Autodesk Fusion 360 part; units mm, degrees
sketch "Sketch1" plane through (0, 0, 0) normal (0, 0, 1) x (1, 0, 0)
  line L0 (0, 0) -> (20.646, 0)
  line L1 (20.646, 0) -> (20.646, 50)
  line L2 (20.646, 50) -> (0, 50)
  line L3 (0, 50) -> (0, 0)
  dimension "d1" = 20.646
  dimension "d2" = 50
extrude "Extrude1" add sketch "Sketch1" along normal blind 5
sketch "Sketch2" plane through (0, 0, 5) normal (0, 0, 1) x (-1, 0, 0)
  line L0 (0, -50) -> (0, 0)
  line L1 (0, 0) -> (-20.646, 0)
  line L2 (-20.646, 0) -> (-20.646, -50)
  line L3 (-20.646, -50) -> (0, -50)
sketch "Sketch3" plane through (0, 0, 5) normal (0, 0, 1) x (-1, 0, 0)
  line L0 (-20.646, 0) -> (-20.646, -50)
  line L1 (0, -50) -> (0, 0)
  circle A0 centre (-10.323, -25) radius 8.0085
  dimension "d5" = 16.017
extrude "Extrude2" cut sketch "Sketch3" against normal blind 10
sketch "Sketch4" plane through (0, 0, 5) normal (0, 0, 1) x (-1, 0, 0)
  circle A0 centre (-10.323, -25) radius 8.0085
  line L0 (-10.323, -25) -> (-2.3221, -33.0009)
  line L1 (-10.323, -25) -> (-2.3221, -16.9991)
  line L2 (-10.323, -25) -> (-18.3239, -16.9991)
  line L3 (-10.323, -25) -> (-18.3239, -33.0009)
hole "Hole1" at (2.3221, 16.9991, 5) at (2.3221, 33.0009, 5) at (18.3239, 33.0009, 5) at (18.3239, 16.9991, 5) direction (0, 0, -1) diameter 1.623 depth 16 tip angle 180 counterbore diameter 3.9 counterbore depth 1
sketch "Sketch5" plane through (0, 0, 5) normal (0, 0, 1) x (-1, 0, 0)
  circle A0 centre (-2.3221, -33.0009) radius 1.95
  line L0 (-2.3221, -33.0009) -> (-2.3221, -44.0009)
  circle A1 centre (-18.3239, -33.0009) radius 1.95
  line L1 (-18.3239, -33.0009) -> (-18.3239, -44.0009)
  circle A2 centre (-2.3221, -16.9991) radius 1.95
  line L2 (-2.3221, -16.9991) -> (-2.3221, -5.9991)
  circle A3 centre (-18.3239, -16.9991) radius 1.95
  line L3 (-18.3239, -16.9991) -> (-18.3239, -5.9991)
  dimension "d16" = 11
  dimension "d17" = 11
  dimension "d18" = 11
  dimension "d19" = 11
hole "Hole2" at (2.3221, 5.9991, 5) at (18.3239, 5.9991, 5) at (18.3239, 44.0009, 5) at (2.3221, 44.0009, 5) direction (0, 0, -1) diameter 1.623 end through all counterbore diameter 3.9 counterbore depth 1
sketch "Sketch6" plane through (0, 0, 5) normal (0, 0, 1) x (-1, 0, 0)
Here's how the part is built. I have some questions about the finished solid (model axes, mm). A direction names the side the tool comes from. Give positions to 0.01 mm unless a question says otherwise; leave off trailing zeros. Write each loop counter-clockwise with the first axis right and the second up, starting at its lowest first coordinate (ties: lowest second). Pieces come first, ordered by that corner, then holes.
(1) If I drill on L1, parallel to Y at x = 10.5, z = 4.7; L2, parallel to X at y = 33.5, z = 0.3; L3, parallel to Y at x = 1.25, z = 4.2, over which ranges is the centre line in solid material (lowest first)?
Output values:
L1: y = 0 to 16.99, 33.01 to 50
L2: x = 0 to 1.68, 2.96 to 17.68, 18.96 to 20.65
L3: y = 0 to 4.37, 7.63 to 15.37, 18.63 to 31.37, 34.63 to 42.37, 45.63 to 50
(2) On a 3-axis mill with a long thin cutter (end or side, diameter ignored), from which of +Z, -Z, +X, -X, +Y, -Y can I reach the whole of each face in a straight line? I mean faces 4 (the face through (2, 32, 4)), 5 (the face through (18.82, 17.64, 1.97)). Say none if no direction works.
Output values:
face 4: +Z
face 5: +Z, -Z
(3) Imagine slicing it at B-B, the plane z = 1.1. Count the separate pieces of the cut face and the enclosed holes in it, and give its area (3 significant figures).
Output values:
separate pieces: 1
enclosed holes: 9
area: 814 mm2
(4) Thinking about a two-plate mould opening in Y: for faces 1 (the face through (2, 43, 4)), 2 (the face through (10, 50, 2)), 3 (the face through (10, 0, 2)), which applies, pulls with the +Y half, pulls with the -Y half, needs draft (parallel to the pull), parting line crosses it, or undercut?
Output values:
face 1: undercut
face 2: pulls with the +Y half
face 3: pulls with the -Y half
(5) Imagine slicing it at A-A, the plane y = 25. Write out the boundary of the cut face in (x, z).
Output values:
outline: (0, 0) - (2.31, 0) - (2.31, 5) - (0, 5) - close; (18.33, 0) - (20.65, 0) - (20.65, 5) - (18.33, 5) - close
(6) Will these pins go through, and if not, where does the flat tip stop? pin 1 (2.5 mm diameter, centred on x = 18.32, y = 44, fed in from +Z); pin 2 (1 mm diameter, centred on x = 2.32, y = 17, fed in from -Z).
Output values:
pin 1: stops at z = 4
pin 2: passes through
(7) Imagine slicing it at C-C, the plane x = 9.5. Write out the boundary of the cut face in (y, z).
Output values:
outline: (0, 0) - (17.03, 0) - (17.03, 5) - (0, 5) - close; (32.97, 0) - (50, 0) - (50, 5) - (32.97, 5) - close
